from build123d import *

# Parameters (mm, degrees)
SKETCH_1_R      = 42.5
EXTRUDE_1_DEPTH = 20
SKETCH_2_R      = 37.5
EXTRUDE_2_DEPTH = 30
SKETCH_3_R      = 24
EXTRUDE_3_DEPTH = 93


with BuildPart() as part:
    # ｽｹｯﾁ1 → ﾎﾞｽ - 押し出し1 (new body)
    with BuildSketch(Plane.XY):
        Circle(SKETCH_1_R)
    extrude(amount=EXTRUDE_1_DEPTH)

    # ｽｹｯﾁ2 → ﾎﾞｽ - 押し出し2 (add)
    with BuildSketch(Plane.XY.offset(20)):
        Circle(SKETCH_2_R)
    extrude(amount=EXTRUDE_2_DEPTH)

    # ｽｹｯﾁ3 → ﾎﾞｽ - 押し出し3 (add)
    with BuildSketch(Plane.XY.offset(50)):
        with Locations((0, 5)):
            Circle(SKETCH_3_R)
    extrude(amount=EXTRUDE_3_DEPTH)


solid = part.part
Geometry check sheet. Reference: the model listing, model coordinates, mm. A direction names the side the tool comes from. Give positions to 0.01 mm unless a question says otherwise; leave off trailing zeros. Loops run counter-clockwise (first coordinate to the right, second up) from the corner with the lowest first, then second, coordinate; pieces in that order, holes last. Notation, with made-up numbers: (58.5, -7) -> (109.5, -7) arc R22 ccw to (109.5, 22) -> close; hole circle Ø4 at (-20, -26). An arc over 180 degrees is marked (long way). Answer in a Markdown table with one row per item. Add a question column.
1) Cross-section at A-A on x = 0. Record the boundary of the cut face in (y, z).
2) Material ranges on probe 1 along Z at (x, y) = (24.5, -23.5); probe 2 along Z at (x, y) = (26.5, 32); probe 3 along Y at (x, z) = (26, 35.5), recorded low to high. Write a range as from..to.
3) Cross-section at C-C on z = 39.5. Record the boundary of the cut face in (x, y), and give its area (3 significant figures).
4) Gauge pin test, flat ends, axial feed: P1, Ø1, axis at x = 7, z = 56, coming from the -Y side; P2, Ø2, axis at x = 8.5, z = 83, coming from the -Y side; P3, Ø12, axis at y = 19.5, z = 64, coming from the -X side. Record the tip position at first contact, or that the pin passes through.
5) Set-up check for faces 1 (the face through (0, 5, 143)), 2 (the face through (-23.977, 6.055, 95.849)): record each of +Z, -Z, +X, -X, +Y, -Y from which the full face is reachable in a straight line by a thin tool's end or side.
6) Cross-section at B-B on y = 34. Record the boundary of the cut face in (x, z), and give its area (3 significant figures).
7) Cross-section at D-D on x = 16. Record the boundary of the cut face in (y, z).
Outcome:
| question | item | result |
|---|---|---|
| 1 | outline | (-42.5, 0) -> (42.5, 0) -> (42.5, 20) -> (37.5, 20) -> (37.5, 50) -> (29, 50) -> (29, 143) -> (-19, 143) -> (-19, 50) -> (-37.5, 50) -> (-37.5, 20) -> (-42.5, 20) -> close |
| 2 | probe 1 | z = 0..50 |
| 2 | probe 2 | z = 0..20 |
| 2 | probe 3 | y = -27.02..27.02 |
| 3 | outline | circle Ø75 at (0, 0) |
| 3 | area | 4,420 mm^2 |
| 4 | P1 | stops at y = -18.1 |
| 4 | P2 | stops at y = -17.8 |
| 4 | P3 | stops at x = -22.44 |
| 5 | face 1 | +Z, +X, -X, +Y, -Y |
| 5 | face 2 | +Z |
| 6 | outline | (-25.5, 0) -> (25.5, 0) -> (25.5, 20) -> (15.82, 20) -> (15.82, 50) -> (-15.82, 50) -> (-15.82, 20) -> (-25.5, 20) -> close |
| 6 | area | 1,970 mm^2 |
| 7 | outline | (-39.37, 0) -> (39.37, 0) -> (39.37, 20) -> (33.92, 20) -> (33.92, 50) -> (22.89, 50) -> (22.89, 143) -> (-12.89, 143) -> (-12.89, 50) -> (-33.92, 50) -> (-33.92, 20) -> (-39.37, 20) -> close |
